Check sheet for the modelled part. Datum: model origin and axes. Units: mm. Face numbers are marked on the shaded views. A direction names the side the tool comes from. Round coordinates to 2 decimals unless told otherwise and drop trailing zeros. Write each loop counter-clockwise with the first axis right and the second up, starting at its lowest first coordinate (ties: lowest second). Pieces come first, ordered by that corner, then holes. Notation, with made-up numbers: (87.5, 80) - (108.5, 80) arc R22 cw to (108.5, 110) - close; hole circle Ø4 at (36, -11.5). An arc over 180 degrees is marked (long way). Answer as a JSON object with one key per item and string values. Group by question number.
Item 1: Sectioned sample at A-A on y = 114. Record the boundary of the cut face in (x, z) (3 decimals), plus the area to 3 significant figures.
Item 2: Gauge pin test, flat ends, axial feed: P1, Ø3, axis at y = 66.5, z = -52, coming from the -X side (3 decimals); P2, Ø4, axis at y = 103, z = -39, coming from the +X side (3 decimals); P3, Ø10, axis at x = 252, z = -82.5, coming from the -Y side. Record the tip position at first contact, or that the pin passes through.
Item 3: Thickness scan on line 1 (X direction, y = 219, z = -42.5) (3 decimals); line 2 (X direction, y = 88.5, z = -44.5) (3 decimals); line 3 (Z direction, x = -303, y = 134). Record the ranges inside material, lowest first.
Item 4: Sectioned sample at C-C on x = 21. Record the boundary of the cut face in (y, z), plus the area to 3 significant figures.
Item 5: Sectioned sample at D-D on x = -267.5. Record the boundary of the cut face in (y, z).
Item 6: Release check for a two-part mould opening along X. For the marked faces 5, 6, 7 and 8 record: pulls with the +X half, pulls with the -X half, needs draft (parallel to the pull), parting line crosses it, or undercut.
Item 7: Sectioned sample at B-B on z = -16.5. Record the boundary of the cut face in (x, y) (3 decimals), plus the area to 3 significant figures.
Item 8: Set-up check for the marked faces 1, 2, 3 and 4: record each of +Z, -Z, +X, -X, +Y, -Y from which the full face is reachable in a straight line by a thin tool's end or side.
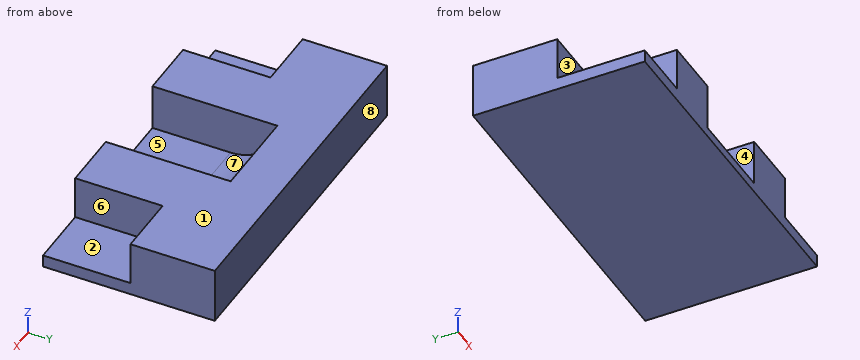
```python
from build123d import *

# Parameters (mm, degrees)
SKETCH1_W           = 679.45
SKETCH1_H           = 114.3
BOSS_EXTRUDE1_DEPTH = 349.25
SKETCH4_W           = 184.15
SKETCH4_H           = 95.25
SKETCH5_W           = 127
SKETCH5_H           = 88.9
CUT_EXTRUDE1_DEPTH  = 177.8


with BuildPart() as part:
    # Sketch1 → Boss-Extrude1 (new body)
    with BuildSketch(Plane(origin=(0, 0, 0), x_dir=(1, 0, 0), z_dir=(0, 1, 0))):
        with Locations((0, 57.15)):
            Rectangle(SKETCH1_W, SKETCH1_H)
    extrude(amount=BOSS_EXTRUDE1_DEPTH)

    # Cut-Sweep4: sweep along a path in Sketch2
    with BuildLine(Plane(origin=(0, 0, 0), x_dir=(0, 0, -1), z_dir=(1, 0, 0))) as cut_sweep4_path:
        Line((47.625, 0), (47.625, 158.75))
        ThreePointArc((47.625, 158.75), (33.675960454, 192.425960454), (0, 206.375))
        Line((0, 206.375), (-25.4, 206.375))
    # Sketch4 → Cut-Sweep4 (sweep, cut)
    with BuildSketch(Plane(origin=(0, 0, 0), x_dir=(1, 0, 0), z_dir=(0, 1, 0))):
        with Locations((0, 47.625)):
            Rectangle(SKETCH4_W, SKETCH4_H)
    sweep(path=cut_sweep4_path.line, mode=Mode.SUBTRACT)

    # Sketch5 → Cut-Extrude1 (cut)
    with BuildSketch(Plane(origin=(0, 0, 0), x_dir=(1, 0, 0), z_dir=(0, 1, 0))):
        with Locations((-276.225, 44.45)):
            Rectangle(SKETCH5_W, SKETCH5_H)
        with Locations((276.225, 44.45)):
            Rectangle(SKETCH5_W, SKETCH5_H)
    extrude(amount=CUT_EXTRUDE1_DEPTH, mode=Mode.SUBTRACT)


solid = part.part
```
Completed:
{
 "1": {"outline": "(-339.725, -114.3) - (339.725, -114.3) - (339.725, -88.9) - (212.725, -88.9) - (212.725, 0) - (92.075, 0) - (92.075, -95.25) - (-92.075, -95.25) - (-92.075, 0) - (-212.725, 0) - (-212.725, -88.9) - (-339.725, -88.9) - close", "area": "37,500 mm²"},
 "2": {"P1": "x = -212.725", "P2": "x = 212.725", "P3": "y = 177.8"},
 "3": {"line 1": "-339.725 to -92.075, 92.075 to 339.725", "line 2": "-212.725 to -92.075, 92.075 to 212.725", "line 3": "-114.3 to -88.9"},
 "4": {"outline": "(0, -114.3) - (349.25, -114.3) - (349.25, 0) - (254, 0) arc R95.25 cw to (158.75, -95.25) - (0, -95.25) - close", "area": "17,700 mm²"},
 "5": {"outline": "(0, -114.3) - (349.25, -114.3) - (349.25, 0) - (177.8, 0) - (177.8, -88.9) - (0, -88.9) - close"},
 "6": {"face 5": "undercut", "face 6": "pulls with the +X half", "face 7": "undercut", "face 8": "needs draft"},
 "7": {"outline": "(-339.725, 177.8) - (-212.725, 177.8) - (-212.725, 0) - (-92.075, 0) - (-92.075, 252.56) - (92.075, 252.56) - (92.075, 0) - (212.725, 0) - (212.725, 177.8) - (339.725, 177.8) - (339.725, 349.25) - (-339.725, 349.25) - close", "area": "146,000 mm²"},
 "8": {"face 1": "+Z, +X, -X, +Y, -Y", "face 2": "+Z, +X, -Y", "face 3": "+Z, -X, -Y", "face 4": "+Z, -Y"}
}
